Can you work these out from the model? Positions are in its coordinate system, mm. Give positions to 0.01 mm unless a question says otherwise; leave off trailing zeros. Loops run counter-clockwise (first coordinate to the right, second up) from the corner with the lowest first, then second, coordinate; pieces in that order, holes last. Notation, with made-up numbers: M -14,75.25 L 21,75.25 A5 cw 21,84.25 Z; hole C 5,28.25 d6. An arc over 180 degrees is marked long. Put each result on its own line as item: value. Start each with the question number.
1) Please list where these lines run through material, in increasing order: line 1 along Y through (x, z) = (1.4, -232.5); line 2 along Y through (x, z) = (7, -295); line 3 along Z through (x, y) = (1, 34). Write a range as from..to.
2) If we mould it in two halves opening along Z, with no side actions, what happens to faces 1 (the flat face through (2, -10, -104)), 2 (the flat face through (0.986, -2.628, -31.587)), 3 (the flat face through (6, 27, -325.5)), 4 (the flat face through (0.986, -9.914, -47.694))? For each: +Z half, -Z half, draft (parallel to the pull), parting line (faces both ways), or undercut.
3) Imagine slicing it at B-B (z = -232.5). Write out the boundary of the cut face in (x, y), then the cut area to 3 significant figures.
4) Imagine slicing it at A-A (x = 8.5). Write out the boundary of the cut face in (y, z), then the cut area to 3 significant figures.
5) Imagine slicing it at C-C (y = -36.5). Write out the boundary of the cut face in (x, z), then the cut area to 3 significant figures.
6) For P1, Ø5, axis at x = 2.5, y = -5, coming from the +Z side; P2, Ø2, axis at x = 0.5, y = -40.5, coming from the -Z side; P3, Ø5, axis at x = 6, y = 46, coming from the -Z side, each with a flat end and sliding along its axis, tell me the tip position at first contact or that it passes through.
from build123d import *

# Parameters (mm, degrees)
SKETCH_1_W      = 2
SKETCH_1_H      = 40
SKETCH_1_W_2    = 40
SKETCH_1_H_2    = 2
SKETCH_1_W_3    = 50
SKETCH_1_R      = 15
SKETCH_1_W_4    = 30
EXTRUDE_3_DEPTH = 2
SKETCH_2_W      = 174.5
SKETCH_2_H      = 6
EXTRUDE_4_DEPTH = 10


with BuildPart() as part:
    # 草图1 → 凸台-拉伸3 (new body)
    with BuildSketch(Plane(origin=(0, 0, 0), x_dir=(0, 0, -1), z_dir=(1, 0, 0))):
        with BuildLine():
            Line((350, 50), (0, 50))
            ThreePointArc((0, 50), (-50, 0), (0, -50))
            Line((0, -50), (350, -50))
            Line((350, -50), (350, -20))
            Line((350, -20), (352, -20))
            Line((352, -20), (352, 20))
            Line((352, 20), (350, 20))
            Line((350, 20), (350, 50))
        make_face()
        with BuildLine():
            ThreePointArc((145, 38), (146.757359313, 42.242640687), (151, 44))
            Line((151, 44), (325.5, 44))
            ThreePointArc((325.5, 44), (329.742640687, 42.242640687), (331.5, 38))
            Line((331.5, 38), (331.5, 30))
            Line((331.5, 30), (151, 30))
            ThreePointArc((151, 30), (146.757359313, 31.757359313), (145, 36))
            Line((145, 36), (145, 38))
        make_face(mode=Mode.SUBTRACT)
        with Locations((1, 0)):
            Rectangle(SKETCH_1_W, SKETCH_1_H, mode=Mode.SUBTRACT)
        with Locations((60, -41)):
            Rectangle(SKETCH_1_W_2, SKETCH_1_H_2, mode=Mode.SUBTRACT)
        with BuildLine():
            Line((97.931678324, -20), (32.068321676, -20))
            ThreePointArc((32.068321676, -20), (30.600998265, -18.811387231), (31.459113977, -17.129282677))
            Line((31.459113977, -17.129282677), (64.390792301, -2.4929812))
            ThreePointArc((64.390792301, -2.4929812), (65, -2.363698523), (65.609207699, -2.4929812))
            Line((65.609207699, -2.4929812), (98.540886023, -17.129282677))
            ThreePointArc((98.540886023, -17.129282677), (99.399001735, -18.811387231), (97.931678324, -20))
        make_face(mode=Mode.SUBTRACT)
        with BuildLine():
            Line((135, -17.39868764), (135, 7.388444501))
            ThreePointArc((135, 7.388444501), (135.75290891, 8.68915773), (137.255806538, 8.684112853))
            Line((137.255806538, 8.684112853), (158.585016393, -3.757926229))
            ThreePointArc((158.585016393, -3.757926229), (159.329207689, -5.056143052), (158.580609404, -6.35182365))
            Line((158.580609404, -6.35182365), (137.25139955, -18.69691671))
            ThreePointArc((137.25139955, -18.69691671), (135.750700102, -18.698129698), (135, -17.39868764))
        make_face(mode=Mode.SUBTRACT)
        with Locations((175, -41)):
            Rectangle(SKETCH_1_W_3, SKETCH_1_H_2, mode=Mode.SUBTRACT)
        with Locations((295, -41)):
            Rectangle(SKETCH_1_W_3, SKETCH_1_H_2, mode=Mode.SUBTRACT)
        with BuildLine():
            Line((189.451619145, -25), (145.548380855, -25))
            ThreePointArc((145.548380855, -25), (144.100364535, -23.891469969), (144.792574317, -22.204331649))
            Line((144.792574317, -22.204331649), (166.744193462, -9.399220481))
            ThreePointArc((166.744193462, -9.399220481), (167.5, -9.194888832), (168.255806538, -9.399220481))
            Line((168.255806538, -9.399220481), (190.207425683, -22.204331649))
            ThreePointArc((190.207425683, -22.204331649), (190.899635465, -23.891469969), (189.451619145, -25))
        make_face(mode=Mode.SUBTRACT)
        with BuildLine():
            ThreePointArc((197.744193462, 8.684112853), (199.24709109, 8.68915773), (200, 7.388444501))
            Line((200, 7.388444501), (200, -17.388444501))
            ThreePointArc((200, -17.388444501), (199.24709109, -18.68915773), (197.744193462, -18.684112853))
            Line((197.744193462, -18.684112853), (176.506860031, -6.295668351))
            ThreePointArc((176.506860031, -6.295668351), (175.762666569, -5), (176.506860031, -3.704331649))
            Line((176.506860031, -3.704331649), (197.744193462, 8.684112853))
        make_face(mode=Mode.SUBTRACT)
        with Locations((232.5, -5)):
            Circle(SKETCH_1_R, mode=Mode.SUBTRACT)
        with BuildLine():
            Line((319.974166797, -25.394327939), (276.070928507, -25.394327939))
            ThreePointArc((276.070928507, -25.394327939), (274.622912187, -24.285797907), (275.315121969, -22.598659587))
            Line((275.315121969, -22.598659587), (297.266741114, -9.793548419))
            ThreePointArc((297.266741114, -9.793548419), (298.022547652, -9.589216771), (298.778354191, -9.793548419))
            Line((298.778354191, -9.793548419), (320.729973336, -22.598659587))
            ThreePointArc((320.729973336, -22.598659587), (321.422183118, -24.285797907), (319.974166797, -25.394327939))
        make_face(mode=Mode.SUBTRACT)
        with BuildLine():
            Line((265.522547652, -17.793015579), (265.522547652, 6.994116563))
            ThreePointArc((265.522547652, 6.994116563), (266.275456563, 8.294829792), (267.778354191, 8.289784914))
            Line((267.778354191, 8.289784914), (289.107564045, -4.152254168))
            ThreePointArc((289.107564045, -4.152254168), (289.851755342, -5.45047099), (289.103157056, -6.746151588))
            Line((289.103157056, -6.746151588), (267.773947202, -19.091244648))
            ThreePointArc((267.773947202, -19.091244648), (266.273247754, -19.092457637), (265.522547652, -17.793015579))
        make_face(mode=Mode.SUBTRACT)
        with BuildLine():
            ThreePointArc((327.730104505, 8.28146303), (329.239985391, 8.298885363), (330, 6.994116563))
            Line((330, 6.994116563), (330, -17.477952976))
            ThreePointArc((330, -17.477952976), (329.24709109, -18.778666205), (327.744193462, -18.773621327))
            Line((327.744193462, -18.773621327), (307.029407683, -6.68999629))
            ThreePointArc((307.029407683, -6.68999629), (306.285236534, -5.40250951), (307.015318726, -4.106981472))
            Line((307.015318726, -4.106981472), (327.730104505, 8.28146303))
        make_face(mode=Mode.SUBTRACT)
        with BuildLine():
            Line((15, -7.691857033), (15, 17.691857033))
            ThreePointArc((15, 17.691857033), (15.682629689, 18.94959539), (17.109207699, 19.062574356))
            Line((17.109207699, 19.062574356), (45.665886023, 6.370717323))
            ThreePointArc((45.665886023, 6.370717323), (46.556678324, 5), (45.665886023, 3.629282677))
            Line((45.665886023, 3.629282677), (17.109207699, -9.062574356))
            ThreePointArc((17.109207699, -9.062574356), (15.682629689, -8.94959539), (15, -7.691857033))
        make_face(mode=Mode.SUBTRACT)
        with BuildLine():
            Line((112.890792301, -9.062574356), (84.334113977, 3.629282677))
            ThreePointArc((84.334113977, 3.629282677), (83.443321676, 5), (84.334113977, 6.370717323))
            Line((84.334113977, 6.370717323), (112.890792301, 19.062574356))
            ThreePointArc((112.890792301, 19.062574356), (114.317370311, 18.94959539), (115, 17.691857033))
            Line((115, 17.691857033), (115, -7.691857033))
            ThreePointArc((115, -7.691857033), (114.317370311, -8.94959539), (112.890792301, -9.062574356))
        make_face(mode=Mode.SUBTRACT)
        with BuildLine():
            ThreePointArc((31.459113977, 27.129282677), (30.600998265, 28.811387231), (32.068321676, 30))
            Line((32.068321676, 30), (97.931678324, 30))
            ThreePointArc((97.931678324, 30), (99.399001735, 28.811387231), (98.540886023, 27.129282677))
            Line((98.540886023, 27.129282677), (65.609207699, 12.4929812))
            ThreePointArc((65.609207699, 12.4929812), (65, 12.363698523), (64.390792301, 12.4929812))
            Line((64.390792301, 12.4929812), (31.459113977, 27.129282677))
        make_face(mode=Mode.SUBTRACT)
        with BuildLine():
            ThreePointArc((144.792574317, 12.204331649), (144.100364535, 13.891469969), (145.548380855, 15))
            Line((145.548380855, 15), (189.885145799, 15))
            ThreePointArc((189.885145799, 15), (191.333825129, 13.889009252), (190.636545348, 12.20177093))
            Line((190.636545348, 12.20177093), (168.381459159, -0.679208343))
            ThreePointArc((168.381459159, -0.679208343), (167.627511138, -0.880977109), (166.874253072, -0.676647625))
            Line((166.874253072, -0.676647625), (144.792574317, 12.204331649))
        make_face(mode=Mode.SUBTRACT)
        with BuildLine():
            ThreePointArc((275.298059327, 12.21443661), (274.625531488, 13.901032988), (276.070928507, 15))
            Line((276.070928507, 15), (321.088992758, 15))
            ThreePointArc((321.088992758, 15), (322.537672089, 13.889009252), (321.840392308, 12.20177093))
            Line((321.840392308, 12.20177093), (298.904006812, -1.073536282))
            ThreePointArc((298.904006812, -1.073536282), (298.140143671, -1.275255431), (297.379738082, -1.060870603))
            Line((297.379738082, -1.060870603), (275.298059327, 12.21443661))
        make_face(mode=Mode.SUBTRACT)
        Polygon((-40, 20), (-9.698170842, 42.091834457), (-8.519939671, 40.475736902), (-38.821768829, 18.383902445), align=None, mode=Mode.SUBTRACT)
        with Locations((-25, -9)):
            Rectangle(SKETCH_1_W_4, SKETCH_1_H_2, mode=Mode.SUBTRACT)
        Polygon((-40, -20), (-38.821768829, -18.383902445), (-8.519939671, -40.475736902), (-9.698170842, -42.091834457), align=None, mode=Mode.SUBTRACT)
    extrude(amount=EXTRUDE_3_DEPTH)

    # 草图2 → 凸台-拉伸4 (add)
    with BuildSketch(Plane(origin=(0, 0, 0), x_dir=(0, 0, -1), z_dir=(1, 0, 0))):
        with Locations((238.25, 47)):
            Rectangle(SKETCH_2_W, SKETCH_2_H)
        Polygon((151, 30), (151, 24), (325.5, 23.560383637), (325.5, 30), align=None)
    extrude(amount=EXTRUDE_4_DEPTH)


solid = part.part
Recorded:
1. line 1: -50..-20, 10..30, 44..50
1. line 2: 23.64..30, 44..50
1. line 3: -350..-331.5, -145.34..17.4, 20.8..36.66
2. face 1: draft
2. face 2: undercut
2. face 3: -Z half
2. face 4: undercut
3. outline: M 0,-50 L 2,-50 L 2,-20 L 0,-20 Z; M 0,10 L 2,10 L 2,23.79 L 10,23.79 L 10,30 L 0,30 Z; M 0,44 L 10,44 L 10,50 L 0,50 Z
3. area: 210 mm²
4. outline: M 23.56,-325.5 L 30,-325.5 L 30,-151 L 24,-151 Z; M 44,-325.5 L 50,-325.5 L 50,-151 L 44,-151 Z
4. area: 2,130 mm²
5. outline: M 0,-350 L 2,-350 L 2,13.97 L 0,13.97 Z; M 0,17.37 L 2,17.37 L 2,34.17 L 0,34.17 Z
5. area: 762 mm²
6. P1: z = 49.93
6. P2: z = -350
6. P3: z = -325.5
